Work out the finished part from the listing and answer in its coordinate system (mm). Face numbers are marked on the shaded views. Round coordinates to 2 decimals unless told otherwise and drop trailing zeros. Loops run counter-clockwise (first coordinate to the right, second up) from the corner with the lowest first, then second, coordinate; pieces in that order, holes last.
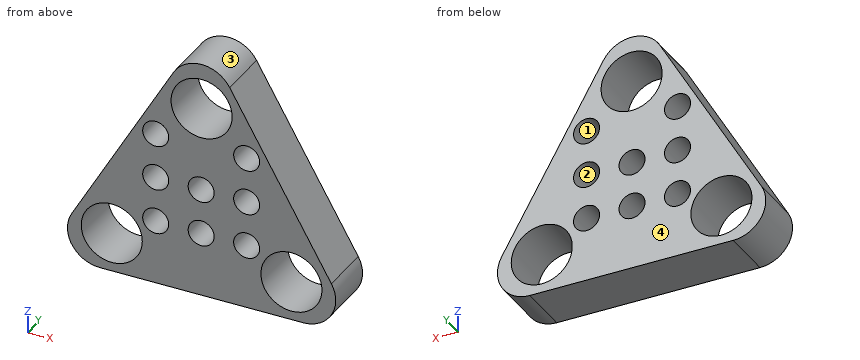
```python
from build123d import *

# Parameters (mm, degrees)
SKETCH1_R      = 2.35
SKETCH1_R_2    = 1
EXTRUDE1_DEPTH = 4


with BuildPart() as part:
    # Sketch1 → Extrude1 (new body)
    with BuildSketch(Plane(origin=(0, 0, 0), x_dir=(1, 0, 0), z_dir=(0, 1, 0))):
        with BuildLine():
            Line((-5.186041147, 3.316192399), (2.637731834, -10.234979911))
            ThreePointArc((2.637731834, -10.234979911), (4.802795343, -11.484979911), (6.967858853, -10.234979911))
            Line((6.967858853, -10.234979911), (14.791631834, 3.316192399))
            ThreePointArc((14.791631834, 3.316192399), (14.791631834, 5.816192399), (12.626568324, 7.066192399))
            Line((12.626568324, 7.066192399), (-3.020977638, 7.066192399))
            ThreePointArc((-3.020977638, 7.066192399), (-5.186041147, 5.816192399), (-5.186041147, 3.316192399))
        make_face()
        with Locations((-2.110635714, 4.040606244)):
            Circle(SKETCH1_R, mode=Mode.SUBTRACT)
        with Locations((4.802795343, -7.933807601)):
            Circle(SKETCH1_R, mode=Mode.SUBTRACT)
        with Locations((11.7162264, 4.040606244)):
            Circle(SKETCH1_R, mode=Mode.SUBTRACT)
        with Locations((1.270334632, 2.088602105)):
            Circle(SKETCH1_R_2, mode=Mode.SUBTRACT)
        with Locations((4.770334632, 2.088602105)):
            Circle(SKETCH1_R_2, mode=Mode.SUBTRACT)
        with Locations((8.270334632, 2.088602105)):
            Circle(SKETCH1_R_2, mode=Mode.SUBTRACT)
        with Locations((1.270334632, -1.411397895)):
            Circle(SKETCH1_R_2, mode=Mode.SUBTRACT)
        with Locations((4.770334632, -1.411397895)):
            Circle(SKETCH1_R_2, mode=Mode.SUBTRACT)
        with Locations((8.270334632, -1.411397895)):
            Circle(SKETCH1_R_2, mode=Mode.SUBTRACT)
        with Locations((1.270334632, -4.911397895)):
            Circle(SKETCH1_R_2, mode=Mode.SUBTRACT)
        with Locations((8.270334632, -4.911397895)):
            Circle(SKETCH1_R_2, mode=Mode.SUBTRACT)
    extrude(amount=EXTRUDE1_DEPTH)


solid = part.part
```
1. Find section C-C (x = 5.5). Write down the section's boundary in (y, z), then the cut area to 3 significant figures.
Answer key:
outline: (0, -7.07) - (4, -7.07) - (4, -2.77) - (0, -2.77) - close; (0, -1.4) - (4, -1.4) - (4, 0.73) - (0, 0.73) - close; (0, 2.1) - (4, 2.1) - (4, 5.69) - (0, 5.69) - close; (0, 10.18) - (4, 10.18) - (4, 11.39) - (0, 11.39) - close
area: 44.9 mm2
2. Find section A-A (z = -4.75). Write down the section's boundary in (x, y).
Answer key:
outline: (-5.51, 0) - (-4.35, 0) - (-4.35, 4) - (-5.51, 4) - close; (0.13, 0) - (9.48, 0) - (9.48, 4) - (0.13, 4) - close; (13.96, 0) - (15.12, 0) - (15.12, 4) - (13.96, 4) - close
3. Given pin 1 (3 mm diameter, centred on x = 4.77, z = -2.09, fed in from -Y); pin 2 (4 mm diameter, centred on x = -2.11, z = -4.04, fed in from -Y); pin 3 (2 mm diameter, centred on y = 1.5, z = -2, fed in from +X), each flat-ended and moving along its own axis, determine where each tip first touches the part or whether it passes through.
Answer key:
pin 1: stops at y = 0
pin 2: passes through
pin 3: stops at x = 14.61
4. Find section D-D (z = 8.75). Write down the section's boundary in (x, y), then the cut area to 3 significant figures.
Answer key:
outline: (1.78, 0) - (2.6, 0) - (2.6, 4) - (1.78, 4) - close; (7.01, 0) - (7.83, 0) - (7.83, 4) - (7.01, 4) - close
area: 6.55 mm2
5. Find section B-B (y = 1.1). Give the number of separate pieces and of enclosed holes in the cut face, then the cut area to 3 significant figures.
Answer key:
separate pieces: 1
enclosed holes: 11
area: 166 mm2
6. Consider probe 1 along Z at (x, y) = (1.5, 3.2); probe 2 along Z at (x, y) = (2, 2.65); probe 3 along X at (y, z) = (2.55, -3). Determine where each line is inside the solid, lowest interval first.
Answer key:
probe 1: z = -7.07 to -3.06, -1.12 to 0.44, 2.38 to 3.94, 5.88 to 8.26
probe 2: z = -7.07 to -2.77, -1.4 to 0.73, 2.1 to 4.23, 5.6 to 9.13
probe 3: x = -5 to -4.22, 0 to 0.86, 1.68 to 4.36, 5.18 to 7.86, 8.68 to 9.61, 13.82 to 14.61
7. Determine the mould class of the marked faces 1, 2, 3 and 4 for opening direction Z: +Z half, -Z half, draft (parallel to the pull), parting line (faces both ways), or undercut.
Answer key:
face 1: undercut
face 2: undercut
face 3: +Z half
face 4: draft
